Could you check a few things on this model? Use its own coordinates, in mm. A direction names the side the tool comes from. Round coordinates to 2 decimals unless told otherwise and drop trailing zeros. Loops run counter-clockwise (first coordinate to the right, second up) from the corner with the lowest first, then second, coordinate; pieces in that order, holes last. Notation, with made-up numbers: (58, 69.5) -> (114, 69.5) arc R26 ccw to (114, 99.5) -> close; hole circle Ø9 at (37, -26). An arc over 180 degrees is marked (long way). One line per item, written item: value.
```python
from build123d import *

# Parameters (mm, degrees)
ESBO_O1_W                = 100.3
ESBO_O1_H                = 45.3
ESBO_O1_R                = 5.15
ESBO_O1_W_2              = 5.6
ESBO_O1_H_2              = 4.1
RESSALTO_EXTRUS_O1_DEPTH = 7
ESBO_O2_R                = 1.65
CORTE_EXTRUS_O1_DEPTH    = 35
FILETE1_R                = 10
FILETE2_R                = 30


with BuildPart() as part:
    # Esboço1 → Ressalto-extrusão1 (new body)
    with BuildSketch(Plane.XY):
        with Locations((0.087398189, -8.941132561)):
            Rectangle(ESBO_O1_W, ESBO_O1_H)
        with Locations((-16.508590221, 3.558867439)):
            Circle(ESBO_O1_R, mode=Mode.SUBTRACT)
        with Locations((16.491409779, 3.558867439)):
            Circle(ESBO_O1_R, mode=Mode.SUBTRACT)
        with Locations((-39.912601811, -21.441132561)):
            Circle(ESBO_O1_R, mode=Mode.SUBTRACT)
        with Locations((40.087398189, -21.441132561)):
            Circle(ESBO_O1_R, mode=Mode.SUBTRACT)
        with Locations((-5.635596016, -11.291132561)):
            Rectangle(ESBO_O1_W_2, ESBO_O1_H_2, mode=Mode.SUBTRACT)
        with Locations((5.810392394, -11.291132561)):
            Rectangle(ESBO_O1_W_2, ESBO_O1_H_2, mode=Mode.SUBTRACT)
    extrude(amount=RESSALTO_EXTRUS_O1_DEPTH)

    # Esboço2 → Corte-extrusão1 (cut)
    with BuildSketch(Plane(origin=(0, 13.708867439, 0), x_dir=(1, 0, 0), z_dir=(0, 1, 0))):
        with Locations(Location((-5.722601811, -3.5, 0), (0, 0, 180))):
            Circle(ESBO_O2_R)
        with Locations(Location((5.897398189, -3.5, 0), (0, 0, 270))):
            Circle(ESBO_O2_R)
    extrude(amount=-CORTE_EXTRUS_O1_DEPTH, mode=Mode.SUBTRACT)

    # Filete1
    filete1_edges = [part.edges().sort_by_distance(p)[0] for p in [
        (50.237398189, -31.591132561, 3.5),
        (-50.062601811, -31.591132561, 3.5),
    ]]
    fillet(filete1_edges, radius=FILETE1_R)

    # Filete2
    filete2_edges = [part.edges().sort_by_distance(p)[0] for p in [
        (-50.062601811, 13.708867439, 3.5),
        (50.237398189, 13.708867439, 3.5),
    ]]
    fillet(filete2_edges, radius=FILETE2_R)


solid = part.part
```
Item 1: If we section it at A-A on x = -37.5: List the corners of the cut face in (y, z) for me, plus the area to 3 significant figures.
Output:
outline: (-31.59, 0) -> (-25.99, 0) -> (-25.99, 7) -> (-31.59, 7) -> close; (-16.89, 0) -> (8.12, 0) -> (8.12, 7) -> (-16.89, 7) -> close
area: 214 mm²
Item 2: If we section it at C-C on y = -15: List the corners of the cut face in (x, z) for me.
Output:
outline: (-50.03, 0) -> (50.21, 0) -> (50.21, 7) -> (-50.03, 7) -> close; hole circle Ø3.3 at (-5.72, 3.5); hole circle Ø3.3 at (5.9, 3.5)
Item 3: If we section it at B-B on y = -22.5: List the corners of the cut face in (x, z) for me.
Output:
outline: (-50.02, 0) -> (-44.95, 0) -> (-44.95, 7) -> (-50.02, 7) -> close; (-34.87, 0) -> (35.05, 0) -> (35.05, 7) -> (-34.87, 7) -> close; (45.13, 0) -> (50.2, 0) -> (50.2, 7) -> (45.13, 7) -> close
Item 4: Will these pins go through, and if not, where does the flat tip stop? pin 1 Ø4 at (y, z) = (1, 3) entering from -X; pin 2 Ø3 at (x, z) = (-5.72, 3.5) entering from +Y; pin 3 Ø4 at (y, z) = (-9, 4.5) entering from +X.
Output:
pin 1: stops at x = -45.87
pin 2: stops at y = -21.29
pin 3: stops at x = 49.77
Item 5: If we mould it in two halves opening along Z, with no side actions, what happens to faces 1 (the face through (-1, -9, 0)), 2 (the face through (4.287, -17.26, 3.142)), 3 (the face through (-41.508, 4.688, 3.549))? For each: released by +Z, released by -Z, zero draft, split by the parting line, or undercut.
Output:
face 1: released by -Z
face 2: undercut
face 3: zero draft
Item 6: If we section it at D-D on x = 42: List the corners of the cut face in (y, z) for me, plus the area to 3 significant figures.
Output:
outline: (-31.43, 0) -> (-26.22, 0) -> (-26.22, 7) -> (-31.43, 7) -> close; (-16.66, 0) -> (4.36, 0) -> (4.36, 7) -> (-16.66, 7) -> close
area: 184 mm²
Item 7: For faces 4 (the face through (-47.211, -28.584, 3.549)), 5 (the face through (-6, -21.291, 4)), 6 (the face through (-8, -9.241, 3)), which set-ups out of +Z, -Z, +X, -X, +Y, -Y let a thin tool reach every point of the face, with its end or its side?
Output:
face 4: +Z, -Z, -X, -Y
face 5: +Y
face 6: +Z, -Z
Item 8: I need wall thicknesses on line 1 (X direction, y = -21, z = 1.5); line 2 (X direction, y = 3.5, z = 4); line 3 (X direction, y = 4, z = 1.5). Which ranges of each line are inside material? Lowest first, please. Write a range as from..to.
Output:
line 1: x = -50.06..-45.04, -34.78..34.96, 45.22..50.24
line 2: x = -42.61..-21.66, -11.36..-7.3, -4.15..4.32, 7.47..11.34, 21.64..42.78
line 3: x = -42.16..-21.64, -11.38..11.36, 21.62..42.33
